For this review, take the finished solid that the model builds, in its own axes (mm). A direction names the side the tool comes from. Coordinates: 2 decimals unless noted, no trailing zeros. Loops run counter-clockwise (first coordinate to the right, second up) from the corner with the lowest first, then second, coordinate; pieces in that order, holes last.
1. Take a section at A-A, the plane x = -27. State the section outline as (y, z) points, then the cut area to 3 significant figures.
2. Take a section at B-B, the plane y = 8.75. State the section outline as (x, z) points.
3. Take a section at C-C, the plane z = 21. State the section outline as (x, y) points.
4. Machinability: for faces 4 (the face through (57.7, -4.52, -0.16)), 5 (the face through (80.207, 9.204, 0.67)), 6 (the face through (79.244, -0.084, 18.078)), 7 (the face through (-4, 0, -12.5)), 8 (the face through (95.969, 0, -34)), which of the approach directions +Z, -Z, +X, -X, +Y, -Y give a long, thin tool a straight path to every point of the face, cutting with its end or side? Answer none if there is none.
5. To check wall thickness, follow probe 1 along X at (y, z) = (6.5, 1); probe 2 along Y at (x, z) = (102, -37); probe 3 along Z at (x, y) = (102, 0). State the ranges of each line that lie inside material, in increasing order.
6. Clearance check with flat-ended pins moving along their axes: P1, Ø23.5, axis at x = 62, z = 16, coming from the +Y side; P2, Ø3, axis at y = -9, z = 9.5, coming from the +X side; P3, Ø12, axis at x = 11.5, y = 7.5, coming from the -Z side. State where each tip first meets the part, or that it passes through.
7. Take a section at D-D, the plane x = -65.5. State the section outline as (y, z) points, then the cut area to 3 significant figures.
8. Mouldability with a two-part tool opening along Z and no side actions: class faces 1 (the face through (57.7, 4.52, 0.16)), 2 (the face through (110.969, 0, 33)), 3 (the face through (-107.293, -0.175, 0.495)) as pulls with the +Z half, pulls with the -Z half, needs draft (parallel to the pull), parting line crosses it, or undercut.
```python
from build123d import *

# Parameters (mm, degrees)
F1_DEPTH  = 12.5
F0_R      = 12.5
F2_DEPTH  = 6
F3_R      = 5.99999
F4_R      = 5.99999
F6_DEPTH  = 3
F8_DEPTH  = 3
F9_R      = 3
F10_DEPTH = 218.2697359261


# Not quite as in the source:
# - a fillet or chamfer is up to 0.001 mm smaller than in the source, because OpenCascade refuses the exact size


with BuildPart() as f1:
    # F0 (on Front) → F1 (new body, symmetric)
    with BuildSketch(Plane.XZ):
        with BuildLine():
            Line((110.9687169417, 24.9881781063), (110.9687169417, 29.9901491338))
            ThreePointArc((110.9687169417, 29.9901491338), (80.1999810155, 2.02996e-05), (110.9686763555, -29.9901501743))
            Line((110.9686763555, -29.9901501743), (110.9686763555, -24.988179355))
            ThreePointArc((110.9686763555, -24.988179355), (85.1999810155, 2.03026e-05), (110.9687169417, 24.9881781063))
        make_face()
    extrude(amount=F1_DEPTH, both=True)



with BuildPart() as f1b:
    # F0 (on Front) → F1, piece 2 (new body, symmetric)
    with BuildSketch(Plane.XZ):
        with BuildLine():
            ThreePointArc((-80.4711318513, 14.8061428082), (-81.3358966232, 15.2609531347), (-82.1796143085, 15.7537117078))
            ThreePointArc((-82.1796143085, 15.7537117078), (-107.3000189845, 0), (-82.1796143085, -15.7537117078))
            ThreePointArc((-82.1796143085, -15.7537117078), (-81.3358966232, -15.2609531347), (-80.4711318513, -14.8061428082))
            ThreePointArc((-80.4711318513, -14.8061428082), (-74.4783753907, -8.455603916), (-72.3000189845, 0))
            ThreePointArc((-72.3000189845, 0), (-74.4783753907, 8.455603916), (-80.4711318513, 14.8061428082))
        make_face()
        with Locations((-89.8000189845, 0)):
            Circle(F0_R, mode=Mode.SUBTRACT)
    extrude(amount=F1_DEPTH, both=True)


with BuildPart() as f1_1:
    add(f1.part)

    add(f1b.part)  # F2 merges F1b
    # F0 (on Front) → F2 (join, symmetric)
    with BuildSketch(Plane.XZ):
        with BuildLine():
            ThreePointArc((-70.6654197961, 12.5), (-75.702042761, 13.0842948024), (-80.4711318513, 14.8061428082))
            ThreePointArc((-80.4711318513, 14.8061428082), (-74.4783753907, 8.455603916), (-72.3000189845, 0))
            ThreePointArc((-72.3000189845, 0), (-74.4783753907, -8.455603916), (-80.4711318513, -14.8061428082))
            ThreePointArc((-80.4711318513, -14.8061428082), (-75.702042761, -13.0842948024), (-70.6654197961, -12.5))
            Line((-70.6654197961, -12.5), (64.4492452955, -12.5))
            ThreePointArc((64.4492452955, -12.5), (79.0647132666, -17.9493308815), (88.9686763555, -30))
            Line((88.9686763555, -30), (95.9686763555, -30))
            Line((95.9686763555, -30), (95.9686763555, -45))
            Line((95.9686763555, -45), (110.9686763555, -45))
            Line((110.9686763555, -45), (110.9686763555, -29.9901501743))
            ThreePointArc((110.9686763555, -29.9901501743), (80.1999810155, 2.02996e-05), (110.9687169417, 29.9901491338))
            Line((110.9687169417, 29.9901491338), (110.9687169417, 45))
            Line((110.9687169417, 45), (95.9687169417, 44.9999957531))
            Line((95.9687169417, 44.9999957531), (95.9687169417, 29.9999957531))
            Line((95.9687169417, 29.9999957531), (88.9687169417, 29.9999957531))
            ThreePointArc((88.9687169417, 29.9999957531), (79.0647357521, 17.9493194217), (64.4492452955, 12.5))
            Line((64.4492452955, 12.5), (-70.6654197961, 12.5))
        make_face()
    extrude(amount=F2_DEPTH, both=True)

    # F3 (radius 6 in the source; OpenCascade refuses exactly that, so slightly less here)
    f3_edges = [f1_1.edges().sort_by_distance(p)[0] for p in [
        (103.468717, -6, 44.999998),
        (103.468717, 6, 44.999998),
    ]]
    fillet(f3_edges, radius=F3_R)

    # F4 (radius 6 in the source; OpenCascade refuses exactly that, so slightly less here)
    f4_edges = [f1_1.edges().sort_by_distance(p)[0] for p in [
        (103.468676, -6, -45),
        (103.468676, 6, -45),
    ]]
    fillet(f4_edges, radius=F4_R)

    # F5 (on face) → F6 (cut)
    with BuildSketch(Plane.XZ.offset(6)):
        with BuildLine():
            Line((50.1999810155, 7.5), (-49.8000189845, 7.5))
            ThreePointArc((-49.8000189845, 7.5), (-57.3000189845, 0), (-49.8000189845, -7.5))
            Line((-49.8000189845, -7.5), (50.1999810155, -7.5))
            ThreePointArc((50.1999810155, -7.5), (57.6999810155, 0), (50.1999810155, 7.5))
        make_face()
    extrude(amount=-F6_DEPTH, mode=Mode.SUBTRACT)

    # F7 (on face) → F8 (cut)
    with BuildSketch(Plane(origin=(0, 6, 0), x_dir=(-1, 0, 0), z_dir=(0, 1, 0))):
        with BuildLine():
            Line((49.8000189845, 7.5), (-50.1999810155, 7.5))
            ThreePointArc((-50.1999810155, 7.5), (-57.6999810155, 0), (-50.1999810155, -7.5))
            Line((-50.1999810155, -7.5), (49.8000189845, -7.5))
            ThreePointArc((49.8000189845, -7.5), (57.3000189845, 0), (49.8000189845, 7.5))
        make_face()
    extrude(amount=-F8_DEPTH, mode=Mode.SUBTRACT)

    # F9 (on face) → F10 (cut, through all)
    with BuildSketch(Plane.YZ.offset(110.9687169417)):
        with Locations((0, 37.5)):
            Circle(F9_R)
        with Locations((0, -37.5)):
            Circle(F9_R)
    extrude(amount=-F10_DEPTH, mode=Mode.SUBTRACT)


solid = f1_1.part
```
Results list:
1. outline: (-6, -12.5) - (6, -12.5) - (6, -7.5) - (3, -7.5) - (3, 7.5) - (6, 7.5) - (6, 12.5) - (-6, 12.5) - (-6, 7.5) - (-3, 7.5) - (-3, -7.5) - (-6, -7.5) - close
1. area: 210 mm2
2. outline: (-82.18, -15.75) arc R22 cw to (-80.47, -14.81) arc R17.5 ccw to (-80.47, 14.81) arc R22 cw to (-82.18, 15.75) arc R17.5 ccw (long way) to start; (110.97, -29.99) - (110.97, -24.99) arc R25 cw (long way) to (110.97, 24.99) - (110.97, 29.99) arc R30 ccw (long way) to start; hole circle Ø25 at (-89.8, 0)
3. outline: (82.69, -6) - (88.78, -6) - (88.78, -12.5) - (96.64, -12.5) - (96.64, 12.5) - (88.78, 12.5) - (88.78, 6) - (82.69, 6) - close
4. face 4: -Y
4. face 5: +Y
4. face 6: +Z, +Y, -Y
4. face 7: -Z, +Y, -Y
4. face 8: -Z, -X, +Y, -Y
5. probe 1: x = -107.27 to -102.26, -77.34 to -72.33, 80.22 to 85.22
5. probe 2: y = -6 to -2.96, 2.96 to 6
5. probe 3: z = -45 to -40.5, -34.5 to -23.62, 23.62 to 34.5, 40.5 to 45
6. P1: stops at y = 6
6. P2: stops at x = 87.75
6. P3: stops at z = -12.5
7. outline: (-6, -12.5) - (6, -12.5) - (6, 12.5) - (-6, 12.5) - close
7. area: 300 mm2
8. face 1: undercut
8. face 2: needs draft
8. face 3: parting line crosses it
